from build123d import *

# Parameters (mm, degrees)
F0_R        = 11.2
F1_DEPTH    = 7
F2_T1_DEPTH = 7.3091738438


# Not quite as in the source:
# - a fillet or chamfer that OpenCascade refuses, or shapes differently, is made with other operations: its cross-section is extruded or revolved along the edge and cut away or added


with BuildPart() as f1:
    # F0 (on Top) → F1 (new body)
    with BuildSketch(Plane.XY):
        with BuildLine():
            ThreePointArc((24.4140649416, -3.1809629834), (13.4871120811, 7.0747385166), (12.5205974964, 22.0294555527))
            ThreePointArc((12.5205974964, 22.0294555527), (1.5158634118, 44.3693332806), (-13.8361222225, 24.7608951415))
            ThreePointArc((-13.8361222225, 24.7608951415), (-13.7078172482, 24.4365570296), (-13.5843298249, 24.1103542803))
            ThreePointArc((-13.5843298249, 24.1103542803), (-13.113174784, 9.1691492017), (-21.7305353918, -3.0457061978))
            ThreePointArc((-21.7305353918, -3.0457061978), (-36.801707194, -25.6538021325), (-9.7868965809, -22.7441236587))
            ThreePointArc((-9.7868965809, -22.7441236587), (-9.6574780237, -22.2857276707), (-9.506618108, -21.8339342105))
            ThreePointArc((-9.506618108, -21.8339342105), (-0.1149775919, -15.1499512762), (9.4355546579, -21.6048620576))
            ThreePointArc((9.4355546579, -21.6048620576), (35.6773528954, -27.6386082592), (24.4140649416, -3.1809629834))
        make_face()
        with Locations((-23.9752419293, -17.876798287)):
            Circle(F0_R, mode=Mode.SUBTRACT)
        Circle(F0_R, mode=Mode.SUBTRACT)
        with Locations((24.0384545177, -18.176259473)):
            Circle(F0_R, mode=Mode.SUBTRACT)
        with Locations((0, 29.7421794385)):
            Circle(F0_R, mode=Mode.SUBTRACT)
    extrude(amount=F1_DEPTH)

    # F2: fillet of radius 1.5 on 1 edges, made by hand

    # F2_s2 → F2_t1 (cut)
    with BuildSketch(Plane.XY.offset(-0.1545869219)):
        with BuildLine():
            ThreePointArc((-9.7727399665, -22.6912544357), (-9.7886409139, -22.7473067601), (-9.8067032425, -22.8027004014))
            Line((-9.8067032425, -22.8027004014), (-9.6647949432, -22.8520369213))
            ThreePointArc((-9.6647949432, -22.8520369213), (-9.6549491563, -22.8224010768), (-9.6447861139, -22.7928747896))
            Line((-9.6447861139, -22.7928747896), (-9.6413873814, -22.7815286112))
            ThreePointArc((-9.6413873814, -22.7815286112), (-9.6346402283, -22.7554279828), (-9.6274353396, -22.7294463591))
            Line((-9.6274353396, -22.7294463591), (-9.7727399665, -22.6912544357))
        make_face()
    extrude(amount=F2_T1_DEPTH, mode=Mode.SUBTRACT)


solid = f1.part
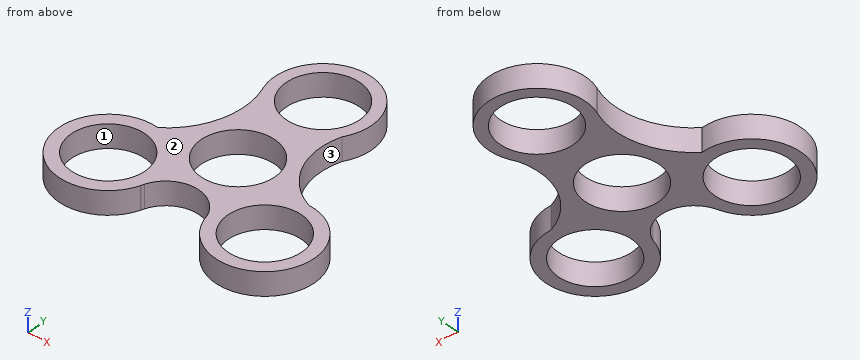
Could you check a few things on this model? Use its own coordinates, in mm. Face numbers are marked on the shaded views. Coordinates: 2 decimals unless noted, no trailing zeros. Order: outer loops, then holes, each group sorted by start corner. A loop starts at its lowest first (then second) coordinate and runs counter-clockwise, first axis right, second up. Notation, with made-up numbers: (20.5, 38) - (27.5, 38) arc R23 ccw to (27.5, 53) - close; hole circle Ø2 at (81.25, -21.75). An arc over 180 degrees is marked (long way). Answer in a Markdown table with one row per item. Add a question column.
(1) If we mould it in two halves opening along X, with no side actions, what happens to the marked faces 1, 2 and 3? For each: released by +X, released by -X, zero draft, split by the parting line, or undercut.
(2) I need wall thicknesses on L1, parallel to Y at x = 0, z = 2; L2, parallel to Y at x = -23.5, z = 2; L3, parallel to X at y = -17.5, z = 6. Which ranges of each line are inside material? Lowest first, please.
(3) If we section it at A-A, the plane x = 0: Please give me the cut outline in (y, z).
(4) If we section it at B-B, the plane x = 27.5: Please give me the cut outline in (y, z).
(5) Will these pins go through, and if not, where does the flat tip stop? pin 1 (3 mm diameter, centred on y = 2.5, z = 4.5, fed in from -X); pin 2 (3 mm diameter, centred on y = -23.5, z = 3.5, fed in from -X); pin 3 (1 mm diameter, centred on x = -26, y = -8, fed in from -Z); pin 4 (3 mm diameter, centred on x = 5.5, z = 5.5, fed in from +Y).
(6) If we section it at C-C, the plane z = 5.75: Please give me the cut outline in (x, y).
(7) If we section it at D-D, the plane y = 0: Please give me the cut outline in (x, z).
Results are:
| question | item | result |
|---|---|---|
| 1 | face 1 | undercut |
| 1 | face 2 | zero draft |
| 1 | face 3 | released by +X |
| 2 | L1 | y = -15.15 to -11.2, 11.2 to 18.54, 40.94 to 44.45 |
| 2 | L2 | y = -32.87 to -29.07, -6.69 to -2.88 |
| 2 | L3 | x = -38.97 to -35.17, -12.78 to -6.47, 6.49 to 12.86, 35.22 to 39.02 |
| 3 | outline | (-15.15, 0) - (-11.2, 0) - (-11.2, 7) - (-15.15, 7) - close; (11.2, 0) - (18.54, 0) - (18.54, 7) - (11.2, 7) - close; (40.94, 0) - (44.45, 0) - (44.45, 7) - (40.94, 7) - close |
| 4 | outline | (-32.77, 0) - (-28.83, 0) - (-28.83, 7) - (-32.77, 7) - close; (-7.52, 0) - (-3.58, 0) - (-3.58, 7) - (-7.52, 7) - close |
| 5 | pin 1 | stops at x = -17.46 |
| 5 | pin 2 | stops at x = -38.4 |
| 5 | pin 3 | passes through |
| 5 | pin 4 | stops at y = 43.89 |
| 6 | outline | (-21.73, -3.05) arc R15 ccw (long way) to (-9.8, -22.77) arc R1.5 ccw to (-9.78, -22.72) arc R10.11 cw to (9.44, -21.6) arc R15 ccw (long way) to (24.41, -3.18) arc R20.39 cw to (12.52, 22.03) arc R14.71 ccw (long way) to (-13.84, 24.76) arc R23.55 cw to start; hole circle Ø22.4 at (-23.98, -17.88); hole circle Ø22.4 at (0, 0); hole circle Ø22.4 at (0, 29.74); hole circle Ø22.4 at (24.04, -18.18) |
| 7 | outline | (-18.33, 0) - (-11.2, 0) - (-11.2, 7) - (-18.33, 7) - close; (11.2, 0) - (19.01, 0) - (19.01, 7) - (11.2, 7) - close |
